Can you work these out from the model? Positions are in its coordinate system, mm. A direction names the side the tool comes from. Coordinates: 2 decimals unless noted, no trailing zeros. Write each question's results on one line, items separated by ' | '. Start each with the question number.
```python
from build123d import *

# Parameters (mm, degrees)
SKETCH004_R     = 75
SKETCH004_R_2   = 2.2
PAD003_DEPTH    = 7
SKETCH005_R     = 5
POCKET001_DEPTH = 4
CHAMFER003_SIZE = 1


with BuildPart() as part:
    # Sketch004 → Pad003 (new body)
    with BuildSketch(Plane.XY):
        Circle(SKETCH004_R)
        Circle(SKETCH004_R_2, mode=Mode.SUBTRACT)
        with Locations((0, 67.5)):
            Circle(SKETCH004_R_2, mode=Mode.SUBTRACT)
        with Locations((0, -67.5)):
            Circle(SKETCH004_R_2, mode=Mode.SUBTRACT)
        with BuildLine():
            ThreePointArc((58.816005, 2), (-58.85, 0), (58.816005, -2))
            Line((58.816005, -2), (6, -2))
            ThreePointArc((6, 2), (-6.324555, 0), (6, -2))
            Line((6, 2), (58.816005, 2))
        make_face(mode=Mode.SUBTRACT)
    extrude(amount=PAD003_DEPTH)

    # Sketch005 (on Face10 of Pad003) → Pocket001 (cut)
    with BuildSketch(Plane.XY.offset(7)):
        with Locations((0, 67.5)):
            Circle(SKETCH005_R)
        with Locations((0, -67.5)):
            Circle(SKETCH005_R)
    extrude(amount=-POCKET001_DEPTH, mode=Mode.SUBTRACT)

    # Chamfer003
    chamfer003_edges = [part.edges().sort_by_distance(p)[0] for p in [
        (-75, 0, 7),
        (-5, -67.5, 7),
        (32.408003, 2, 7),
        (-6.324555, 0, 7),
        (-58.85, 0, 7),
        (32.408003, -2, 7),
        (-2.2, 0, 7),
        (-5, 67.5, 7),
        (-75, 0, 0),
        (32.408003, 2, 0),
        (-58.85, 0, 0),
        (32.408003, -2, 0),
        (-6.324555, 0, 0),
        (-2.2, -67.5, 0),
        (-2.2, 67.5, 0),
        (-2.2, 0, 0),
    ]]
    chamfer(chamfer003_edges, length=CHAMFER003_SIZE)


solid = part.part
```
Q1. If we section it at A-A (x = 32.5): Count the separate pieces of the cut face and the enclosed holes in it, then the cut area to 3 significant figures.
Q2. I'm going to push flat-ended pins straight in: pin 1 Ø16 at (x, y) = (0, 67.5) entering from -Z; pin 2 Ø2 at (y, z) = (39.5, 4) entering from -X; pin 3 Ø3.5 at (x, y) = (0, 0) entering from -Z; pin 4 Ø5.5 at (x, y) = (0, -67.5) entering from +Z. Where does each tip first touch, or does it pass through?
Q3. For faces 4 (the face through (-0.651, -62.543, 4.521)), 5 (the face through (1.183, -65.645, 1.986)), which set-ups out of +Z, -Z, +X, -X, +Y, -Y let a thin tool reach every point of the face, with its end or its side?
Q4. I need wall thicknesses on line 1 along Y through (x, z) = (0, 2.3); line 2 along Y through (x, z) = (0, 3.75); line 3 along Y through (x, z) = (11.5, 5.25). Which ranges of each line are inside material? Lowest first, please. Write a range as from..to.
Q5. Thinking about a two-plate mould opening in X: for faces 1 (the face through (2, 66, 3)), 2 (the face through (0, -5, 7)), 3 (the face through (-9.764, 74.362, 3.465)), which applies, pulls with the +X half, pulls with the -X half, needs draft (parallel to the pull), parting line crosses it, or undercut?
Answer list:
1) separate pieces: 3 | enclosed holes: 0 | area: 281 mm2
2) pin 1: stops at z = 0 | pin 2: stops at x = -64.36 | pin 3: passes through | pin 4: stops at z = 3
3) face 4: +Z | face 5: +Z, -Z
4) line 1: y = -75..-69.7, -65.3..-58.85, -6.32..-2.2, 2.2..6.32, 58.85..65.3, 69.7..75 | line 2: y = -75..-72.5, -62.5..-58.85, -6.32..-2.2, 2.2..6.32, 58.85..62.5, 72.5..75 | line 3: y = -74.11..-57.72, -2..2, 57.72..74.11
5) face 1: undercut | face 2: needs draft | face 3: parting line crosses it
